For this review, take the finished solid that the model builds, in its own axes (mm). Give positions to 0.01 mm unless a question says otherwise; leave off trailing zeros. Write each loop counter-clockwise with the first axis right and the second up, starting at its lowest first coordinate (ties: lowest second). Pieces come first, ordered by that corner, then holes. Notation, with made-up numbers: M -32,-33.5 L -24,-33.5 A23 ccw -24,-21.5 Z; hole C -4,3 d3. An arc over 180 degrees is marked long. One line per item, written item: value. Start each with the question number.
Item 1: Consider section D-D, the plane z = 128.5. Write out the cut boundary in (x, y).
Item 2: Mouldability with a two-part tool opening along X and no side actions: class faces 1 (the face through (190.62, -3.13, 69.5)), 2 (the face through (-4, -6.35, 58)) as released by +X, released by -X, zero draft, split by the parting line, or undercut.
Item 3: Consider section B-B, the plane y = -3.25. Give the number of separate pieces and of enclosed holes in the cut face, and give its area (3 significant figures).
Item 4: Consider section C-C, the plane z = 97. Write out the cut boundary in (x, y).
Item 5: Consider section A-A, the plane x = 13. Write out the cut boundary in (y, z) (3 decimals), and give its area (3 significant figures).
Item 6: To check wall thickness, follow probe 1 along X at (y, z) = (-0.25, 27); probe 2 along Z at (x, y) = (-211, -6) (3 decimals); probe 3 along Z at (x, y) = (-218, -0.25) (3 decimals). State the ranges of each line that lie inside material, in increasing order.
```python
from build123d import *

# Parameters (mm, degrees)
F0_W      = 520.7
F0_H      = 146.05
F0_R      = 31.877
F1_DEPTH  = 6.35
F2_DEPTH  = 6.35
F3_R      = 10.0959291711
F3_R_2    = 9.3516208714
F3_R_3    = 9.399866871
F4_DEPTH  = 25.4
F5_R      = 2.413
F6_DEPTH  = 25.4
F7_W      = 6.35
F7_H      = 6.35
F8_DEPTH  = 25.4
F9_W      = 50.8
F9_H      = 31.75
F10_DEPTH = 25.4
F11_R     = 12.7
F12_DEPTH = 12.7


# Not quite as in the source:
# - a feature names something its author has since deleted; it is built from what else it names


with BuildPart() as f1:
    # F0 (on Front) → F1 (new body)
    with BuildSketch(Plane.XZ):
        with Locations((0.0123051805, 73.0250019237)):
            Rectangle(F0_W, F0_H)
        with Locations((-215.8876948195, 88.9000019237)):
            Circle(F0_R, mode=Mode.SUBTRACT)
        with BuildLine():
            ThreePointArc((-155.9332892075, 49.5438408284), (-145.5947264636, 134.7931724118), (-73.0126948195, 88.9000019237))
            ThreePointArc((-73.0126948195, 88.9000019237), (-77.9195243313, 67.1179702796), (-91.6921004315, 49.5438408284))
            ThreePointArc((-91.6921004315, 49.5438408284), (-123.8126948195, 38.1000019237), (-155.9332892075, 49.5438408284))
        make_face(mode=Mode.SUBTRACT)
        with Locations((-31.7376948195, 88.9000019237)):
            Circle(F0_R, mode=Mode.SUBTRACT)
        with Locations((50.8123051805, 88.9000019237)):
            Circle(F0_R, mode=Mode.SUBTRACT)
        with Locations((133.3623051805, 88.9000019237)):
            Circle(F0_R, mode=Mode.SUBTRACT)
        with Locations((215.9123051805, 88.9000019237)):
            Circle(F0_R, mode=Mode.SUBTRACT)
    extrude(amount=F1_DEPTH)

    # F0 (on Front) → F2 (join)
    with BuildSketch(Plane.XZ):
        with BuildLine():
            Line((-91.6921004315, 49.5438408284), (-155.9332892075, 49.5438408284))
            ThreePointArc((-155.9332892075, 49.5438408284), (-123.8126948195, 38.1000019237), (-91.6921004315, 49.5438408284))
        make_face()
    extrude(amount=F2_DEPTH)

    # F3 (on face) → F4 (cut)
    with BuildSketch(Plane.XZ.offset(6.35)):
        with Locations((-215.8876948195, 25.4000019237)):
            Circle(F3_R)
        with Locations((9.5373051805, 25.4000019237)):
            Circle(F3_R_2)
        with Locations((174.6373051805, 25.4000019237)):
            Circle(F3_R_3)
    extrude(amount=-F4_DEPTH, mode=Mode.SUBTRACT)

    # F5 (on face) → F6 (cut)
    with BuildSketch(Plane.XZ.offset(6.35)):
        with Locations((-155.5626948195, 120.6500019237)):
            Circle(F5_R)
        with Locations((-92.0626948195, 120.6500019237)):
            Circle(F5_R)
        with Locations((-92.0626948195, 57.1500019237)):
            Circle(F5_R)
        with Locations((-155.5626948195, 57.1500019237)):
            Circle(F5_R)
    extrude(amount=-F6_DEPTH, mode=Mode.SUBTRACT)

    # F7 (on face) → F8 (cut)
    with BuildSketch(Plane.XZ.offset(6.35)):
        with Locations((-269.875, 142.875)):
            Rectangle(F7_W, F7_H)
        with Locations((269.875, 142.875)):
            Rectangle(F7_W, F7_H)
    extrude(amount=-F8_DEPTH, mode=Mode.SUBTRACT)

    # F9 (on face) → F10 (cut)
    with BuildSketch(Plane.XZ.offset(6.35)):
        with Locations((-215.8876948195, 25.4000019237)):
            Rectangle(F9_W, F9_H)
        with Locations((9.5373051805, 25.4000019237)):
            Rectangle(F9_W, F9_H)
        with Locations((174.6373051805, 25.4000019237)):
            Rectangle(F9_W, F9_H)
    extrude(amount=-F10_DEPTH, mode=Mode.SUBTRACT)

    # F11 (on face) → F12 (cut, symmetric)
    with BuildSketch(Plane.XZ.offset(6.35)):
        with Locations((-123.8126948195, 25.4000019237)):
            Circle(F11_R)
    extrude(amount=F12_DEPTH, both=True, mode=Mode.SUBTRACT)


solid = f1.part
```
Model answer:
1. outline: M -260.34,-6.35 L -155.63,-6.35 L -155.63,0 L -260.34,0 Z; M -91.99,-6.35 L 260.36,-6.35 L 260.36,0 L -91.99,0 Z
2. face 1: undercut
2. face 2: zero draft
3. separate pieces: 1
3. enclosed holes: 10
3. area: 47,100 mm2
4. outline: M -260.34,-6.35 L -246.72,-6.35 L -246.72,0 L -260.34,0 Z; M -185.06,-6.35 L -173.96,-6.35 L -173.96,0 L -185.06,0 Z; M -73.66,-6.35 L -62.57,-6.35 L -62.57,0 L -73.66,0 Z; M -0.91,-6.35 L 19.98,-6.35 L 19.98,0 L -0.91,0 Z; M 81.64,-6.35 L 102.53,-6.35 L 102.53,0 L 81.64,0 Z; M 164.19,-6.35 L 185.08,-6.35 L 185.08,0 L 164.19,0 Z; M 246.74,-6.35 L 260.36,-6.35 L 260.36,0 L 246.74,0 Z
5. outline: M -6.35,0 L 0,0 L 0,9.525 L -6.35,9.525 Z; M -6.35,41.275 L 0,41.275 L 0,146.05 L -6.35,146.05 Z
5. area: 726 mm2
6. probe 1: x = -260.34 to -241.29, -190.49 to -136.41, -111.21 to -15.86, 34.94 to 149.24, 200.04 to 260.36
6. probe 2: z = 0 to 9.525, 41.275 to 57.4, 120.4 to 146.05
6. probe 3: z = 0 to 9.525, 41.275 to 57.093, 120.707 to 146.05
